Autodesk Inventor part; units mm, degrees
ref_plane "YZ Plane" through (0, 0, 0) normal (1, 0, 0) x (0, 1, 0)
ref_plane "XZ Plane" through (0, 0, 0) normal (0, 1, 0) x (-1, 0, 0)
ref_plane "XY Plane" through (0, 0, 0) normal (0, 0, 1) x (1, 0, 0)
sketch "Sketch1" plane through (0, 0, 0) normal (0, 0, 1) x (1, 0, 0)
  circle A0 centre (0, 0) radius 15
  dimension "d0" = 30
extrude "Extrusion1" add sketch "Sketch1" along normal blind 10
sketch "Sketch2" plane through (0, 0, 10) normal (0, 0, 1) x (1, 0, 0)
  line L0 (-13, -20) -> (13, -20)
  line L1 (13, -20) -> (13, 20)
  line L2 (13, 20) -> (-13, 20)
  line L3 (-13, 20) -> (-13, -20)
  line L4 (-13, -20) -> (13, 20) construction
  line L5 (13, -20) -> (-13, 20) construction
  point P0 (0, 0)
  dimension "d3" = 26
  dimension "d4" = 40
extrude "Extrusion2" cut sketch "Sketch2" against normal blind 10 keep common part
sketch "Sketch3" plane through (0, 0, 10) normal (0, 0, 1) x (1, 0, 0)
  circle A0 centre (0, 0) radius 12
  dimension "d7" = 24
extrude "Extrusion3" add sketch "Sketch3" along normal blind 22
chamfer "Chamfer1" distance 2 angle 45 1 edges at (-12, 0, 32)
sketch "Sketch4" plane through (0, 0, 32) normal (0, 0, 1) x (1, 0, 0)
  line L0 (-7, -7) -> (7, -7)
  line L1 (7, -7) -> (7, 7)
  line L2 (7, 7) -> (-7, 7)
  line L3 (-7, 7) -> (-7, -7)
  line L4 (-7, -7) -> (7, 7) construction
  line L5 (7, -7) -> (-7, 7) construction
  point P0 (0, 0)
  dimension "d13" = 14
extrude "Extrusion4" add sketch "Sketch4" along normal blind 18
thread "Thread1"
properties part number "lab10_2"
The listing builds one solid part. Answer for the finished solid, in the listing's coordinates (mm). A direction names the side the tool comes from. Coordinates: 2 decimals unless noted, no trailing zeros. Write each loop counter-clockwise with the first axis right and the second up, starting at its lowest first coordinate (ties: lowest second). Pieces come first, ordered by that corner, then holes. Notation, with made-up numbers: (-32.5, 40) - (-18.5, 40) arc R19 cw to (-18.5, 48) - close; hole circle Ø8 at (26.25, 28.5). An arc over 180 degrees is marked (long way). One line per item, written item: value.
1) Consider line 1 along X through (y, z) = (-5.25, 38.5); line 2 along Y through (x, z) = (0.25, 8.5). Determine where each line is inside the solid, lowest interval first. Write a range as from..to.
Geometry check:
line 1: x = -7..7
line 2: y = -15..15
2) Each of these flat-tipped pins is pushed along its axis until it touches: pin 1 Ø10 at (y, z) = (9, 17.5) entering from -X; pin 2 Ø11 at (x, z) = (-2, 38.5) entering from +Y; pin 3 Ø10 at (y, z) = (-3, 38) entering from -X. Where does it stop, or does it pass through?
Geometry check:
pin 1: stops at x = -11.31
pin 2: stops at y = 7
pin 3: stops at x = -7
3) A tool of negligible diameter and unlimited length cuts with its end or side. For faces 1 (the flat face through (0, -7, 41)), 2 (the cylindrical face through (-11.99, -0.53, 19.86)), 3 (the flat face through (-7, 0, 41)), 4 (the flat face through (7, 0, 41)), 5 (the flat face through (0, 7, 41)), from which of +Z, -Z, +X, -X, +Y, -Y can it reach the whole face along a straight path? Write none if from no direction.
Geometry check:
face 1: +Z, +X, -X, -Y
face 2: +Z
face 3: +Z, -X, +Y, -Y
face 4: +Z, +X, +Y, -Y
face 5: +Z, +X, -X, +Y
4) Find section C-C (z = 47). Give the vertices of the cut face in (x, y), and give its area (3 significant figures).
Geometry check:
outline: (-7, -7) - (7, -7) - (7, 7) - (-7, 7) - close
area: 196 mm2
5) Find section D-D (z = 22.5). Give the vertices of the cut face in (x, y).
Geometry check:
outline: circle Ø24 at (0, 0)
6) Find section A-A (y = 0). Give the vertices of the cut face in (x, z), and give its area (3 significant figures).
Geometry check:
outline: (-13, 0) - (13, 0) - (13, 10) - (12, 10) - (12, 30) - (10, 32) - (7, 32) - (7, 50) - (-7, 50) - (-7, 32) - (-10, 32) - (-12, 30) - (-12, 10) - (-13, 10) - close
area: 1,040 mm2
7) Find section B-B (x = 0). Give the vertices of the cut face in (y, z), and give its area (3 significant figures).
Geometry check:
outline: (-15, 0) - (15, 0) - (15, 10) - (12, 10) - (12, 30) - (10, 32) - (7, 32) - (7, 50) - (-7, 50) - (-7, 32) - (-10, 32) - (-12, 30) - (-12, 10) - (-15, 10) - close
area: 1,080 mm2
